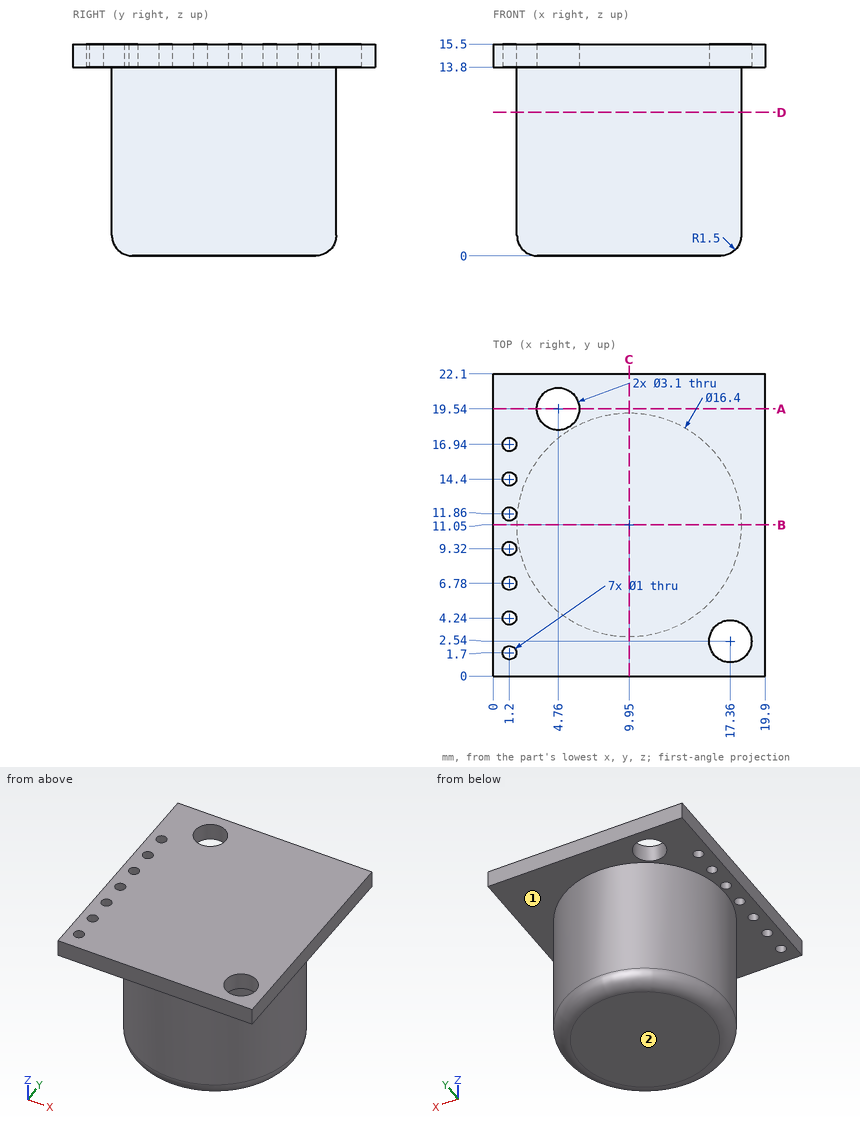
Check sheet for the drawn part. Datum: minimum x, y, z corner. Units: mm. A direction names the side the tool comes from. Give positions to 0.01 mm unless a question says otherwise; leave off trailing zeros. Order: outer loops, then holes, each group sorted by start corner. A loop starts at its lowest first (then second) coordinate and runs counter-clockwise, first axis right, second up.
1. Depth check by flat-ended pin: pin 1 (4 mm diameter, centred on y = 2.5, z = 9.5, fed in from -X); pin 2 (8 mm diameter, centred on x = 13.5, y = 12.5, fed in from -Z); pin 3 (3 mm diameter, centred on x = 7, z = 2.5, fed in from -Y); pin 4 (2.5 mm diameter, centred on x = 17.36, y = 2.54, fed in from +Z). Enter the tip coordinate at first touch or a pass-through.
Completed:
pin 1: stops at x = 5.02
pin 2: stops at z = 0
pin 3: stops at y = 2.98
pin 4: passes through
2. Sectioned sample at B-B (y = 11.05). Record the boundary of the cut face in (x, z).
Completed:
outline: (0, 13.8) - (1.75, 13.8) - (1.75, 1.5) arc R1.5 ccw to (3.25, 0) - (16.65, 0) arc R1.5 ccw to (18.15, 1.5) - (18.15, 13.8) - (19.9, 13.8) - (19.9, 15.5) - (0, 15.5) - close
3. Scan lines: line 1 (Y direction, x = 17.36, z = 14.95); line 2 (Y direction, x = 4.76, z = 14.35); line 3 (Z direction, x = 19, y = 19.25). Record each from-to range of solid material in increasing order.
Completed:
line 1: y = 0 to 0.99, 4.09 to 22.1
line 2: y = 0 to 17.99, 21.09 to 22.1
line 3: z = 13.8 to 15.5
4. Sectioned sample at C-C (x = 9.95). Record the boundary of the cut face in (y, z).
Completed:
outline: (0, 13.8) - (2.85, 13.8) - (2.85, 1.5) arc R1.5 ccw to (4.35, 0) - (17.75, 0) arc R1.5 ccw to (19.25, 1.5) - (19.25, 13.8) - (22.1, 13.8) - (22.1, 15.5) - (0, 15.5) - close
5. Sectioned sample at A-A (y = 19.54). Record the boundary of the cut face in (x, z).
Completed:
outline: (0, 13.8) - (3.21, 13.8) - (3.21, 15.5) - (0, 15.5) - close; (6.31, 13.8) - (19.9, 13.8) - (19.9, 15.5) - (6.31, 15.5) - close
6. Sectioned sample at D-D (z = 10.5). Record the boundary of the cut face in (x, y).
Completed:
outline: circle Ø16.4 at (9.95, 11.05)
7. Access from +Z, -Z, +X, -X, +Y, -Y to the whole of each face (thin tool, end or side, straight path). Record for the marked faces 1 and 2.
Completed:
face 1: -Z
face 2: -Z, +X, -X, +Y, -Y
